The drawing under review shows one solid part. Ordinate dimensions are in mm from its lowest x, y, z. A direction names the side the tool comes from. Round coordinates to 2 decimals unless told otherwise and drop trailing zeros. Order: outer loops, then holes, each group sorted by start corner. A loop starts at its lowest first (then second) coordinate and runs counter-clockwise, first axis right, second up.
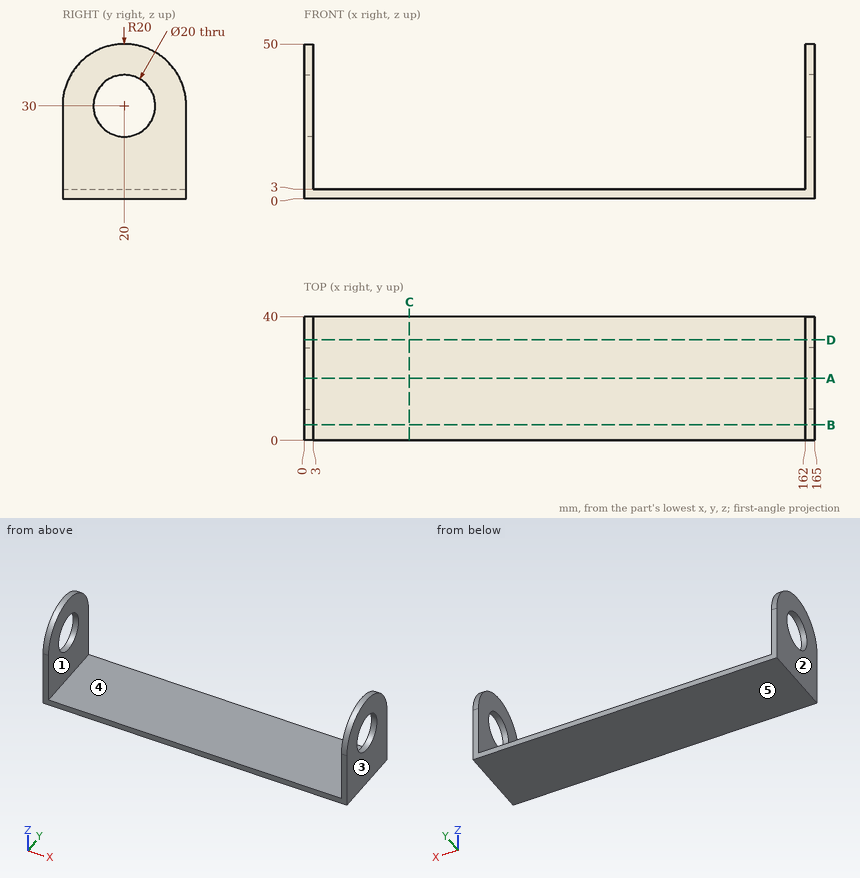
(1) We need section D-D (y = 32.5). Give the boundary of the cut face in (x, z), and give its area (3 significant figures).
(2) We need section A-A (y = 20). Give the boundary of the cut face in (x, z).
(3) We need section C-C (x = 34). Give the boundary of the cut face in (y, z).
(4) The part is to be moulded in two halves that separate along X. For the marked faces 1, 2 and 3, say which applies: pulls with the +X half, pulls with the -X half, needs draft (parallel to the pull), parting line crosses it, or undercut.
(5) Tool access review of the marked faces 4 and 5: name each direction out of +Z, -Z, +X, -X, +Y, -Y from which nothing blocks a thin tool from reaching the whole face with its end or side.
(6) To check wall thickness, follow L1, parallel to Y at x = 2.1, z = 30; L2, parallel to X at y = 31.5, z = 5; L3, parallel to Z at x = 60, y = 18. State the ranges of each line that lie inside material, in increasing order.
(7) Clearance check with flat-ended pins moving along their axes: P1, Ø23, axis at y = 20, z = 30, coming from the +X side; P2, Ø4, axis at x = 120.5, y = 21.5, coming from the +Z side; P3, Ø3, axis at y = 23.5, z = 24, coming from the -X side. State where each tip first meets the part, or that it passes through.
(8) We need section B-B (y = 5). Give the boundary of the cut face in (x, z), and give its area (3 significant figures).
Verdict:
1. outline: (0, 0) - (165, 0) - (165, 45.61) - (162, 45.61) - (162, 3) - (3, 3) - (3, 45.61) - (0, 45.61) - close
1. area: 751 mm2
2. outline: (0, 0) - (165, 0) - (165, 20) - (162, 20) - (162, 3) - (3, 3) - (3, 20) - (0, 20) - close; (0, 40) - (3, 40) - (3, 50) - (0, 50) - close; (162, 40) - (165, 40) - (165, 50) - (162, 50) - close
3. outline: (0, 0) - (40, 0) - (40, 3) - (0, 3) - close
4. face 1: undercut
4. face 2: pulls with the -X half
4. face 3: pulls with the +X half
5. face 4: +Z, +Y, -Y
5. face 5: -Z, +X, -X, +Y, -Y
6. L1: y = 0 to 10, 30 to 40
6. L2: x = 0 to 3, 162 to 165
6. L3: z = 0 to 3
7. P1: stops at x = 165
7. P2: stops at z = 3
7. P3: passes through
8. outline: (0, 0) - (165, 0) - (165, 43.23) - (162, 43.23) - (162, 3) - (3, 3) - (3, 43.23) - (0, 43.23) - close
8. area: 736 mm2
